For this review, take the finished solid that the model builds, in its own axes (mm). A direction names the side the tool comes from. Give positions to 0.01 mm unless a question says otherwise; leave off trailing zeros. Write each loop counter-clockwise with the first axis right and the second up, starting at its lowest first coordinate (ties: lowest second). Pieces come first, ordered by that corner, then holes.
from build123d import *

# Parameters (mm, degrees)
SKETCH1_W           = 63.5
SKETCH1_H           = 111.125
BOSS_EXTRUDE1_DEPTH = 1.5
SKETCH2_W           = 3.175
SKETCH2_H           = 9.525
BOSS_EXTRUDE2_DEPTH = 3
CUT_EXTRUDE1_DEPTH  = 3
FILLET1_R           = 1.5875
SKETCH5_W           = 3
SKETCH5_H           = 6.35
BOSS_EXTRUDE3_DEPTH = 3


with BuildPart() as part:
    # Sketch1 → Boss-Extrude1 (new, symmetric)
    with BuildSketch(Plane(origin=(0, 34.29, 0), x_dir=(1, 0, 0), z_dir=(0, 1, 0))):
        with Locations((0, 120.65)):
            Rectangle(SKETCH1_W, SKETCH1_H)
    extrude(amount=BOSS_EXTRUDE1_DEPTH, both=True)

    # Sketch2 → Boss-Extrude2 (add)
    with BuildSketch(Plane(origin=(0, 35.79, 0), x_dir=(1, 0, 0), z_dir=(0, 1, 0))):
        with Locations((33.3375, 171.45)):
            Rectangle(SKETCH2_W, SKETCH2_H)
        with Locations((-33.3375, 171.45)):
            Rectangle(SKETCH2_W, SKETCH2_H)
        with Locations((33.3375, 120.65)):
            Rectangle(SKETCH2_W, SKETCH2_H)
        with Locations((-33.3375, 120.65)):
            Rectangle(SKETCH2_W, SKETCH2_H)
        with Locations((33.3375, 69.85)):
            Rectangle(SKETCH2_W, SKETCH2_H)
        with Locations((-33.3375, 69.85)):
            Rectangle(SKETCH2_W, SKETCH2_H)
    extrude(amount=-BOSS_EXTRUDE2_DEPTH)

    # Sketch4 → Cut-Extrude1 (cut)
    with BuildSketch(Plane(origin=(0, 35.79, 0), x_dir=(1, 0, 0), z_dir=(0, 1, 0))):
        Polygon((23.118437891, 169.8625), (-23.118437891, 169.8625), (0, 147.466513293), align=None)
        Polygon((-2.281562109, 145.25625), (-25.4, 167.652236707), (-25.4, 122.860263293), align=None)
        Polygon((25.4, 167.652236707), (2.281562109, 145.25625), (25.4, 122.860263293), align=None)
        Polygon((21.479728214, 122.2375), (0, 143.045986707), (-21.479728214, 122.2375), align=None)
        Polygon((-2.281562109, 96.04375), (-25.4, 118.439736707), (-25.4, 73.647763293), align=None)
        Polygon((21.479728214, 119.0625), (-21.479728214, 119.0625), (0, 98.254013293), align=None)
        Polygon((25.4, 73.647763293), (25.4, 118.439736707), (2.281562109, 96.04375), align=None)
        Polygon((23.118437891, 71.4375), (0, 93.833486707), (-23.118437891, 71.4375), align=None)
    extrude(amount=-CUT_EXTRUDE1_DEPTH, mode=Mode.SUBTRACT)

    # Fillet1
    fillet1_edges = [part.edges().sort_by_distance(p)[0] for p in [
        (-21.479728214, 34.29, -119.0625),
        (21.479728214, 34.29, -119.0625),
        (0, 34.29, -98.254013293),
        (-25.4, 34.29, -118.439736707),
        (-2.281562109, 34.29, -96.04375),
        (-25.4, 34.29, -73.647763293),
        (25.4, 34.29, -167.652236707),
        (25.4, 34.29, -122.860263293),
        (2.281562109, 34.29, -145.25625),
        (23.118437891, 34.29, -169.8625),
        (0, 34.29, -147.466513293),
        (-23.118437891, 34.29, -169.8625),
        (2.281562109, 34.29, -96.04375),
        (25.4, 34.29, -118.439736707),
        (25.4, 34.29, -73.647763293),
        (34.925, 34.29, -65.0875),
        (34.925, 34.29, -74.6125),
        (31.75, 34.29, -74.6125),
        (31.75, 34.29, -115.8875),
        (34.925, 34.29, -115.8875),
        (34.925, 34.29, -125.4125),
        (31.75, 34.29, -125.4125),
        (31.75, 34.29, -166.6875),
        (34.925, 34.29, -166.6875),
        (34.925, 34.29, -176.2125),
        (-34.925, 34.29, -166.6875),
        (-31.75, 34.29, -166.6875),
        (-31.75, 34.29, -125.4125),
        (-34.925, 34.29, -125.4125),
        (-34.925, 34.29, -115.8875),
        (-31.75, 34.29, -115.8875),
        (-31.75, 34.29, -74.6125),
        (-34.925, 34.29, -74.6125),
        (-34.925, 34.29, -65.0875),
        (-25.4, 34.29, -122.860263293),
        (-25.4, 34.29, -167.652236707),
        (-2.281562109, 34.29, -145.25625),
        (-23.118437891, 34.29, -71.4375),
        (0, 34.29, -93.833486707),
        (23.118437891, 34.29, -71.4375),
        (-21.479728214, 34.29, -122.2375),
        (0, 34.29, -143.045986707),
        (21.479728214, 34.29, -122.2375),
        (-34.925, 34.29, -176.2125),
    ]]
    fillet(fillet1_edges, radius=FILLET1_R - 0.0001)  # a hair under: the kernel refuses the full size

    # Sketch5 → Boss-Extrude3 (add)
    with BuildSketch(Plane(origin=(0, 35.79, 0), x_dir=(1, 0, 0), z_dir=(0, 1, 0))):
        with Locations((36.425, 171.45)):
            Rectangle(SKETCH5_W, SKETCH5_H)
        with Locations((-36.425, 171.45)):
            Rectangle(SKETCH5_W, SKETCH5_H)
        with Locations((36.425, 120.65)):
            Rectangle(SKETCH5_W, SKETCH5_H)
        with Locations((-36.425, 120.65)):
            Rectangle(SKETCH5_W, SKETCH5_H)
        with Locations((36.425, 69.85)):
            Rectangle(SKETCH5_W, SKETCH5_H)
        with Locations((-36.425, 69.85)):
            Rectangle(SKETCH5_W, SKETCH5_H)
    extrude(amount=-BOSS_EXTRUDE3_DEPTH)


solid = part.part
(1) The part is to be moulded in two halves that separate along X. For faces 1 (the flat face through (37.925, 34, -121)), 2 (the flat face through (25.4, 34, -145)), 3 (the flat face through (0, 34, -176.212)), say which applies: +X half, -X half, draft (parallel to the pull), parting line (faces both ways), or undercut.
(2) We need section D-D (x = -6.5). Write out the cut boundary in (y, z), and give its area (3 significant figures).
(3) We need section B-B (y = 34.55). Count the separate pieces of the cut face and the enclosed holes in it, and give its area (3 significant figures).
(4) We need section C-C (z = -128.5). Write out the cut boundary in (x, y), and give its area (3 significant figures).
(5) We need section A-A (x = 24). Write out the cut boundary in (y, z), and give its area (3 significant figures).
(6) Clearance check with flat-ended pins moving along their axes: pin 1 Ø1.5 at (y, z) = (34, -163.5) entering from -X; pin 2 Ø0.9 at (x, y) = (37, 33.5) entering from -Z (3 decimals); pin 3 Ø0.9 at (x, y) = (-36, 34.5) entering from +Z (3 decimals); pin 4 Ø8 at (x, z) = (1, -86.5) entering from -Y. State where each tip first meets the part, or that it passes through.
(7) Tool access review of faces 4 (the cylindrical face through (-20.66, 34.269, -168.895)), 5 (the flat face through (-36, 34, -123.825)), 6 (the flat face through (-36, 34, -66.675)), 7 (the flat face through (36, 34, -73.025)): name each direction out of +Z, -Z, +X, -X, +Y, -Y from which nothing blocks a thin tool from reaching the whole face with its end or side.
(8) For L1, parallel to Z at x = 24, y = 33.2; L2, parallel to Z at x = 21, y = 34.85; L3, parallel to X at y = 34.25, z = -129, list the stretches that pass through material, from the lowest coordinate up.
The answers:
1. face 1: +X half
1. face 2: undercut
1. face 3: draft
2. outline: (32.79, -176.21) - (35.79, -176.21) - (35.79, -169.86) - (32.79, -169.86) - close; (32.79, -153.76) - (35.79, -153.76) - (35.79, -149.34) - (32.79, -149.34) - close; (32.79, -141.17) - (35.79, -141.17) - (35.79, -136.75) - (32.79, -136.75) - close; (32.79, -122.24) - (35.79, -122.24) - (35.79, -119.06) - (32.79, -119.06) - close; (32.79, -104.55) - (35.79, -104.55) - (35.79, -100.13) - (32.79, -100.13) - close; (32.79, -91.96) - (35.79, -91.96) - (35.79, -87.54) - (32.79, -87.54) - close; (32.79, -71.44) - (35.79, -71.44) - (35.79, -65.09) - (32.79, -65.09) - close
2. area: 101 mm2
3. separate pieces: 1
3. enclosed holes: 8
3. area: 3,400 mm2
4. outline: (-31.75, 32.79) - (-25.4, 32.79) - (-25.4, 35.79) - (-31.75, 35.79) - close; (-19.58, 32.79) - (-15.02, 32.79) - (-15.02, 35.79) - (-19.58, 35.79) - close; (15.02, 32.79) - (19.58, 32.79) - (19.58, 35.79) - (15.02, 35.79) - close; (25.4, 32.79) - (31.75, 32.79) - (31.75, 35.79) - (25.4, 35.79) - close
4. area: 65.5 mm2
5. outline: (32.79, -176.21) - (35.79, -176.21) - (35.79, -165.48) - (32.79, -165.48) - close; (32.79, -125.03) - (35.79, -125.03) - (35.79, -116.27) - (32.79, -116.27) - close; (32.79, -75.82) - (35.79, -75.82) - (35.79, -65.09) - (32.79, -65.09) - close
5. area: 90.7 mm2
6. pin 1: stops at x = -31.75
6. pin 2: stops at z = -174.625
6. pin 3: stops at z = -66.675
6. pin 4: passes through
7. face 4: +Y, -Y
7. face 5: -X, +Y, -Y
7. face 6: +Z, -X, +Y, -Y
7. face 7: +X, +Y, -Y
8. L1: z = -176.21 to -165.48, -125.03 to -116.27, -75.82 to -65.09
8. L2: z = -176.21 to -163.39, -127.12 to -114.18, -77.91 to -65.09
8. L3: x = -31.75 to -25.4, -19.06 to -14.5, 14.5 to 19.06, 25.4 to 31.75
